Study the drawing (mm; zero at the part's minimum x, y, z) and answer. Coordinates: 2 decimals unless noted, no trailing zeros. Order: outer loops, then holes, each group sorted by start corner. A loop starts at its lowest first (then second) coordinate and runs counter-clockwise, first axis right, second up.
1. The part is cut by section D-D, the plane x = 15. Give the vertices of the cut face in (y, z).
2. Find the intervals of material crossed by probe 1 along X at (y, z) = (140, 2.25); probe 2 along Y at (x, z) = (71, 3.5); probe 3 along X at (y, z) = (161.5, 10), in increasing order.
3. The part is cut by section B-B, the plane x = 66.5. Give the vertices of the cut face in (y, z).
4. The part is cut by section C-C, the plane y = 215. Give the vertices of the cut face in (x, z).
5. The part is cut by section A-A, the plane y = 184.5. Give the vertices of the cut face in (x, z).
6. Flat-ended cylindrical pins translate along their axes: pin 1 Ø1.5 at (y, z) = (146, 7.5) entering from -X; pin 2 Ø1 at (y, z) = (196, 10) entering from +X; pin 3 Ø2 at (x, z) = (138, 5) entering from -Y. Find the tip coordinate at first contact, or state that the pin passes through.
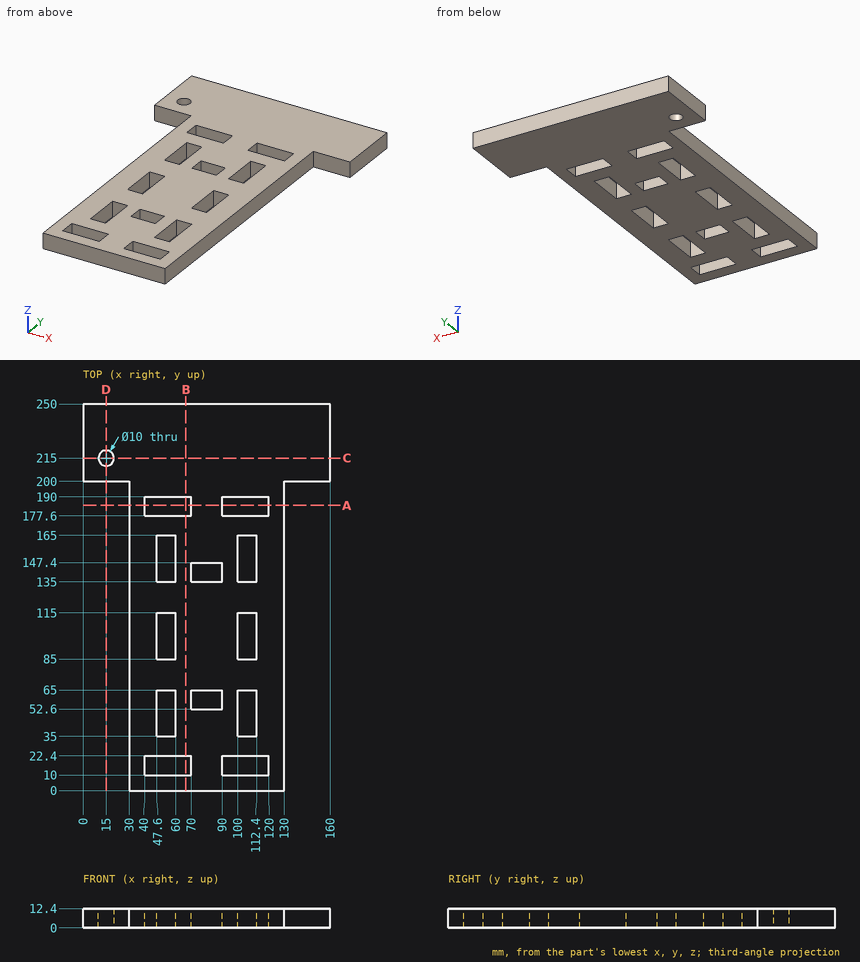
Geometry says:
1. outline: (200, 0) - (210, 0) - (210, 12.4) - (200, 12.4) - close; (220, 0) - (250, 0) - (250, 12.4) - (220, 12.4) - close
2. probe 1: x = 30 to 47.6, 60 to 70, 90 to 100, 112.4 to 130
2. probe 2: y = 0 to 52.6, 65 to 135, 147.4 to 250
2. probe 3: x = 30 to 47.6, 60 to 100, 112.4 to 130
3. outline: (0, 0) - (10, 0) - (10, 12.4) - (0, 12.4) - close; (22.4, 0) - (177.6, 0) - (177.6, 12.4) - (22.4, 12.4) - close; (190, 0) - (250, 0) - (250, 12.4) - (190, 12.4) - close
4. outline: (0, 0) - (10, 0) - (10, 12.4) - (0, 12.4) - close; (20, 0) - (160, 0) - (160, 12.4) - (20, 12.4) - close
5. outline: (30, 0) - (40, 0) - (40, 12.4) - (30, 12.4) - close; (70, 0) - (90, 0) - (90, 12.4) - (70, 12.4) - close; (120, 0) - (130, 0) - (130, 12.4) - (120, 12.4) - close
6. pin 1: stops at x = 30
6. pin 2: stops at x = 130
6. pin 3: stops at y = 200
